```python
from build123d import *

# Parameters (mm, degrees)
EXTRUDE_1_DEPTH      = 110
SKETCH_2_W           = 8
SKETCH_2_H           = 44
CUT_EXTRUDE_3_DEPTH  = 110
CUT_EXTRUDE_4_DEPTH  = 134.373777696
SKETCH_4_R           = 1.75
CUT_EXTRUDE_6_DEPTH  = 10
CUT_EXTRUDE_START    = -2.5
CUT_EXTRUDE_11_DEPTH = 10
SKETCH_6_R           = 2.1
CUT_EXTRUDE_13_DEPTH = 133.388375153


with BuildPart() as part:
    # Эскиз1 → Бобышка-Вытянуть1 (new body)
    with BuildSketch(Plane(origin=(0, 0, 0), x_dir=(1, 0, 0), z_dir=(0, 1, 0))):
        Polygon((-66.825757576, 34.969739794), (-66.825757576, 29.969739794), (-63.825757576, 29.969739794), (-63.825757576, 31.969739794), (-38.825757576, 31.969739794), (-38.825757576, 6.969739794), (-63.825757576, 6.969739794), (-63.825757576, 8.969739794), (-66.825757576, 8.969739794), (-66.825757576, 3.969739794), (-22.123470102, 3.969739794), (-36.579007505, 34.969739794), align=None)
    extrude(amount=EXTRUDE_1_DEPTH)

    # Эскиз2 → Вырез-Вытянуть3 (cut)
    with BuildSketch(Plane(origin=(-16.651582729, 0, 7.764760547), x_dir=(-0.42261826174069383, 0, -0.9063077870366526), z_dir=(0.9063077870366527, 0, -0.4226182617406939))):
        with Locations((16.947588566, 40)):
            Rectangle(SKETCH_2_W, SKETCH_2_H)
    extrude(amount=-CUT_EXTRUDE_3_DEPTH, mode=Mode.SUBTRACT)

    # Эскиз3 → Вырез-Вытянуть4 (cut, through all)
    with BuildSketch(Plane.XZ):
        Polygon((-66.825757576, -3.969739794), (-65.325757576, -8.969739794), (-66.825757576, -8.969739794), align=None)
        Polygon((-66.825757576, -29.969739794), (-66.825757576, -34.969739794), (-65.325757576, -29.969739794), align=None)
    extrude(amount=-CUT_EXTRUDE_4_DEPTH, mode=Mode.SUBTRACT)

    # Эскиз4 → Вырез-Вытянуть6 (cut)
    with BuildSketch(Plane(origin=(-16.651582729, 0, 7.764760547), x_dir=(-0.42261826174069383, 0, -0.9063077870366526), z_dir=(0.9063077870366527, 0, -0.4226182617406939))):
        with Locations((36.747588566, 86.3)):
            Circle(SKETCH_4_R)
        with Locations((36.747588566, 25)):
            Circle(SKETCH_4_R)
    extrude(amount=-CUT_EXTRUDE_6_DEPTH, mode=Mode.SUBTRACT)

    # Эскиз5 → Вырез-Вытянуть11 (cut)
    with BuildSketch(Plane(origin=(-16.651582729, 0, 7.764760547), x_dir=(-0.42261826174069383, 0, -0.9063077870366526), z_dir=(0.9063077870366527, 0, -0.4226182617406939)).offset(CUT_EXTRUDE_START)):
        Polygon((40.78904045, 86.3), (38.768314508, 89.8), (34.726862624, 89.8), (32.706136682, 86.3), (34.726862624, 82.8), (38.768314508, 82.8), align=None)
        Polygon((40.78904045, 25), (38.768314508, 28.5), (34.726862624, 28.5), (32.706136682, 25), (34.726862624, 21.5), (38.768314508, 21.5), align=None)
    extrude(amount=-CUT_EXTRUDE_11_DEPTH, mode=Mode.SUBTRACT)

    # Эскиз6 → Вырез-Вытянуть13 (cut, through all)
    with BuildSketch(Plane.XY.offset(-3.969739794)):
        with Locations((-51.825757576, 94)):
            Circle(SKETCH_6_R)
        with Locations((-51.825757576, 16)):
            Circle(SKETCH_6_R)
    extrude(amount=-CUT_EXTRUDE_13_DEPTH, mode=Mode.SUBTRACT)


solid = part.part
```
Here's how the part is built. I have some questions about the finished solid (model axes, mm). A direction names the side the tool comes from. Coordinates: 2 decimals unless noted, no trailing zeros. Order: outer loops, then holes, each group sorted by start corner. A loop starts at its lowest first (then second) coordinate and runs counter-clockwise, first axis right, second up. Notation, with made-up numbers: M -19,-17 L 10,-17 A19 ccw 10,-2 Z; hole C -28.5,39 d3. An arc over 180 degrees is marked long. Answer as a JSON object with one key per item and string values. Group by question number.
(1) I need wall thicknesses on probe 1 along Z at (x, y) = (-64.5, 83); probe 2 along Z at (x, y) = (-61.5, 42.5); probe 3 along Z at (x, y) = (-31.5, 91). Which ranges of each line are inside material? Lowest first, please.
(2) Suppose I cut it at D-D, the plane z = -19. Please give me the cut outline in (x, y).
(3) Suppose I cut it at A-A, the plane y = 16. Please give me the cut outline in (x, z).
(4) If we mould it in two halves opening along Y, with no side actions, what happens to faces 4 (the face through (-29.25, 54.23, -19.25)), 5 (the face through (-33.203, 26.735, -24.813)), 6 (the face through (-36, 21.5, -24)), 7 (the face through (-38, 0, -18))? For each: released by +Y, released by -Y, zero draft, split by the parting line, or undercut.
(5) Suppose I cut it at C-C, the plane z = -5.5. Please give me the cut outline in (x, y), then the cut area to 3 significant figures.
(6) Which directions (+Z, -Z, +X, -X, +Y, -Y) give clear straight access to the entire face, cutting with the end or side of a thin tool? Please do faces 1 (the face through (-36.17, 88.07, -20.35)), 2 (the face through (-63.826, 54, -8)), 3 (the face through (-37.46, 23.23, -26.41)).
(7) Suppose I cut it at B-B, the plane x = -61. Please give me the cut outline in (y, z), then the cut area to 3 significant figures.
(8) For pin 1 (6 mm diameter, centred on x = -27.5, z = -6.5, fed in from -Y); pin 2 (3 mm diameter, centred on y = 27.5, z = -19.5, fed in from -X); pin 3 (1 mm diameter, centred on x = -38.5, y = 56, fed in from +Z); pin 4 (1.6 mm diameter, centred on y = 62, z = -31.5, fed in from +X), each with a flat end and sliding along its axis, tell me the tip position at first contact or that it passes through.
Values found:
{
 "1": {"probe 1": "z = -34.97 to -29.97, -8.97 to -3.97", "probe 2": "z = -34.97 to -31.97, -6.97 to -3.97", "probe 3": "z = -24.08 to -3.97"},
 "2": {"outline": "M -38.83,0 L -29.13,0 L -29.13,110 L -38.83,110 L -38.83,87.9 L -36.64,86.3 L -38.83,84.7 L -38.83,26.6 L -36.64,25 L -38.83,23.4 Z"},
 "3": {"outline": "M -66.83,-34.97 L -53.93,-34.97 L -53.93,-31.97 L -63.83,-31.97 L -63.83,-29.97 L -65.33,-29.97 Z; M -66.83,-3.97 L -65.33,-8.97 L -63.83,-8.97 L -63.83,-6.97 L -53.93,-6.97 L -53.93,-3.97 Z; M -49.73,-34.97 L -36.58,-34.97 L -22.12,-3.97 L -49.73,-3.97 L -49.73,-6.97 L -38.83,-6.97 L -38.83,-31.97 L -49.73,-31.97 Z"},
 "4": {"face 4": "zero draft", "face 5": "undercut", "face 6": "undercut", "face 7": "released by -Y"},
 "5": {"outline": "M -66.37,0 L -22.84,0 L -22.84,18 L -37.77,18 L -37.77,62 L -22.84,62 L -22.84,110 L -66.37,110 Z; hole C -51.83,16 d4.2; hole C -51.83,94 d4.2", "area": "4,100 mm^2"},
 "6": {"face 1": "-X", "face 2": "+Y, -Y", "face 3": "none"},
 "7": {"outline": "M 0,-34.97 L 110,-34.97 L 110,-31.97 L 0,-31.97 Z; M 0,-6.97 L 110,-6.97 L 110,-3.97 L 0,-3.97 Z", "area": "660 mm^2"},
 "8": {"pin 1": "stops at y = 0", "pin 2": "stops at x = -38.83", "pin 3": "stops at z = -4.93", "pin 4": "stops at x = -34.59"}
}
